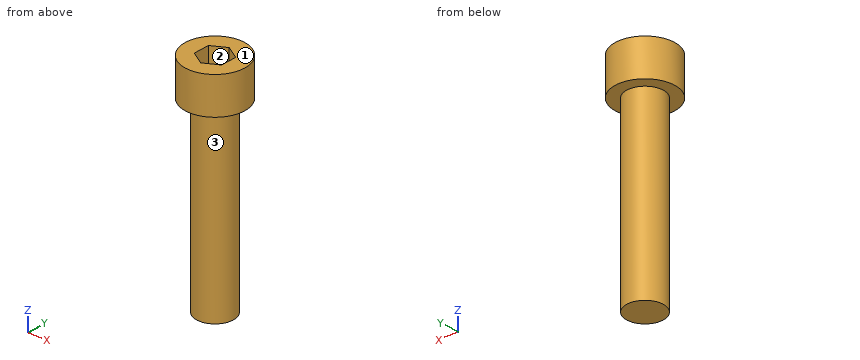
```python
from build123d import *

# Parameters (mm, degrees)
F0_R     = 6.5
F1_DEPTH = 8
F3_DEPTH = 4
F4_R     = 4
F5_DEPTH = 40


with BuildPart() as f1:
    # F0 (on Top) → F1 (new body)
    with BuildSketch(Plane.XY):
        Circle(F0_R)
    extrude(amount=F1_DEPTH)

    # F2 (on face) → F3 (cut)
    with BuildSketch(Plane.XY.offset(8)):
        Polygon((3, 1.732051), (0, 3.464102), (-3, 1.732051), (-3, -1.732051), (0, -3.464102), (3, -1.732051), align=None)
    extrude(amount=-F3_DEPTH, mode=Mode.SUBTRACT)

    # F4 (on face) → F5 (join)
    with BuildSketch(Plane(origin=(0, 0, 0), x_dir=(1, 0, 0), z_dir=(0, 0, -1))):
        Circle(F4_R)
    extrude(amount=F5_DEPTH)


solid = f1.part
```
Here's how the part is built. I have some questions about the finished solid (model axes, mm). Face numbers are marked on the shaded views. Coordinates: 2 decimals unless noted, no trailing zeros. Loops run counter-clockwise (first coordinate to the right, second up) from the corner with the lowest first, then second, coordinate; pieces in that order, holes last. Notation, with made-up numbers: (74, 37.25) -> (113, 37.25) arc R19 cw to (113, 57.25) -> close; hole circle Ø8 at (24.5, -33.5). An arc over 180 degrees is marked (long way). Return JSON: item names as keys, results as strings.
1) If we section it at C-C, the plane z = -11.5: Write out the boundary of the cut face in (x, y), then the cut area to 3 significant figures.
Results below:
{"outline": "circle Ø8 at (0, 0)", "area": "50.3 mm²"}
2) I need wall thicknesses on line 1 (X direction, y = 0, z = -17); line 2 (Z direction, x = -1.25, y = -1.25); line 3 (X direction, y = 3, z = 6). Which ranges of each line are inside material? Lowest first, please. Write a range as from..to.
Results below:
{"line 1": "-4..4", "line 2": "-40..4", "line 3": "-5.77..-0.8, 0.8..5.77"}
3) If we section it at D-D, the plane x = 5: Write out the boundary of the cut face in (y, z).
Results below:
{"outline": "(-4.15, 0) -> (4.15, 0) -> (4.15, 8) -> (-4.15, 8) -> close"}
4) Thinking about a two-plate mould opening in X: for the marked faces 1, 2 and 3, which applies, +X half, -X half, draft (parallel to the pull), parting line (faces both ways), or undercut?
Results below:
{"face 1": "draft", "face 2": "undercut", "face 3": "parting line"}
5) If we section it at B-B, the plane x = -1: Write out the boundary of the cut face in (y, z).
Results below:
{"outline": "(-6.42, 0) -> (-3.87, 0) -> (-3.87, -40) -> (3.87, -40) -> (3.87, 0) -> (6.42, 0) -> (6.42, 8) -> (2.89, 8) -> (2.89, 4) -> (-2.89, 4) -> (-2.89, 8) -> (-6.42, 8) -> close"}
6) Will these pins go through, and if not, where does the flat tip stop? pin 1 (3 mm diameter, centred on y = -3.5, z = -3, fed in from +X); pin 2 (6 mm diameter, centred on y = 4, z = -26.5, fed in from +X); pin 3 (4 mm diameter, centred on x = 0.5, z = -24.5, fed in from +Y).
Results below:
{"pin 1": "x = 3.46", "pin 2": "x = 3.87", "pin 3": "y = 4"}
7) If we section it at A-A, the plane y = 0: Write out the boundary of the cut face in (x, z), then the cut area to 3 significant figures.
Results below:
{"outline": "(-6.5, 0) -> (-4, 0) -> (-4, -40) -> (4, -40) -> (4, 0) -> (6.5, 0) -> (6.5, 8) -> (3, 8) -> (3, 4) -> (-3, 4) -> (-3, 8) -> (-6.5, 8) -> close", "area": "400 mm²"}
